Geometry: see drawing. Coordinates: mm, zero at the bounding-box minimum. A direction names the side the tool comes from. Round coordinates to 2 decimals unless told otherwise and drop trailing zeros. Write each loop counter-clockwise with the first axis right and the second up, starting at its lowest first coordinate (ties: lowest second). Pieces come first, ordered by that corner, then holes. Notation, with made-up numbers: M 13,-20 L 17,-20 A30 cw 17,13 Z; hole C 55,-13.75 d8. An arc over 180 degrees is marked long. Use one line per item in the form item = value. Start each with the question number.
Item 1: Section query D-D (y = 5.5). Return loops of the section in (x, z) (1 decimal), and give its area (3 significant figures).
Item 2: Pin query (flat end, axial travel): pin 1 Ø1.5 at (y, z) = (10.5, 0.5) entering from -X (1 decimal); pin 2 Ø1 at (y, z) = (31, 1) entering from -X. Return the tip coordinate at first contact, or that it passes through.
Item 3: Section query B-B (x = 26). Return loops of the section in (y, z), and give its area (3 significant figures).
Item 4: Section query A-A (y = 35.1). Return loops of the section in (x, z) (1 decimal).
Item 5: Pull-direction query (X, two-part tool) for the marked faces 3, 4 and 5; classes: pulls with the +X half, pulls with the -X half, needs draft (parallel to the pull), parting line crosses it, or undercut.
Item 6: Reachability of the marked faces 1 and 2 from +Z, -Z, +X, -X, +Y, -Y: full face, straight path, thin tool, end or side. Return the list, or none.
Item 7: Ray query, probe 1 along Y at (x, z) = (12, 1.5) (1 decimal); probe 2 along Y at (x, z) = (14, 0.95); probe 3 along X at (y, z) = (22.5, 1.35). Return the intervals inside material, ascending.
Item 8: Section query C-C (z = 0.9). Return loops of the section in (x, y).
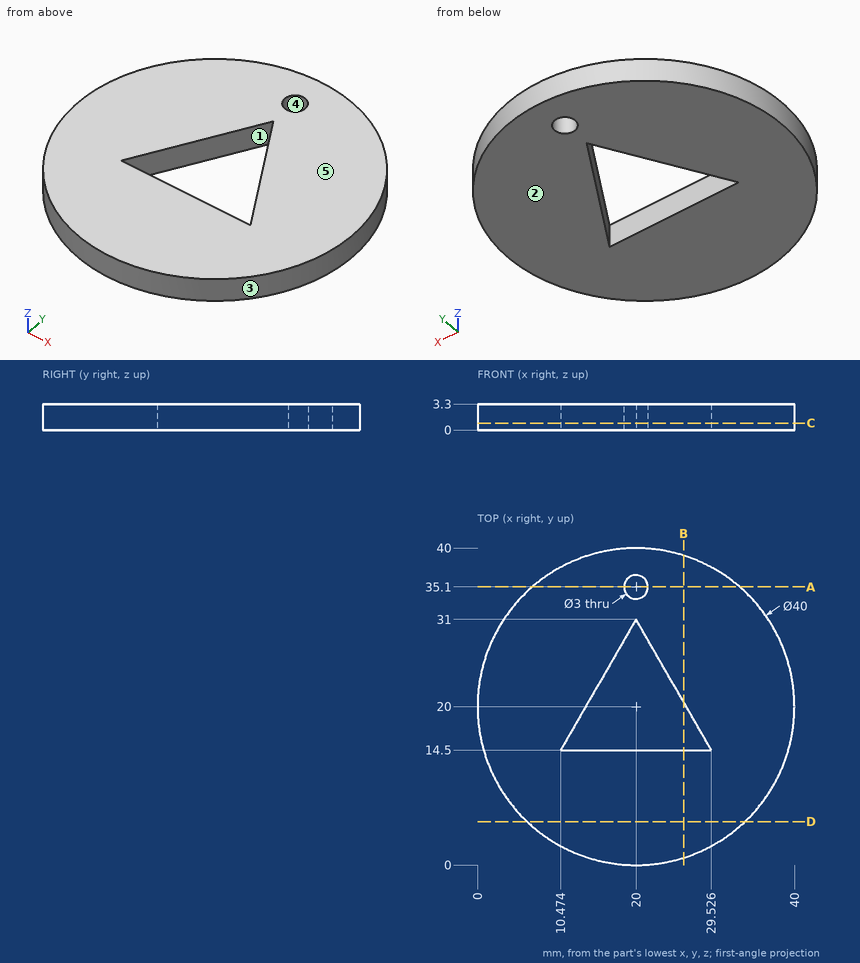
Working result:
q1.outline = M 6.2,0 L 33.8,0 L 33.8,3.3 L 6.2,3.3 Z
q1.area = 90.9 mm²
q2.pin_1 = 2
q2.pin_2 = 2.98
q3.outline = M 0.92,0 L 14.5,0 L 14.5,3.3 L 0.92,3.3 Z; M 20.61,0 L 39.08,0 L 39.08,3.3 L 20.61,3.3 Z
q3.area = 106 mm²
q4.outline = M 6.9,0 L 18.5,0 L 18.5,3.3 L 6.9,3.3 Z; M 21.5,0 L 33.1,0 L 33.1,3.3 L 21.5,3.3 Z
q5.face_3 = parting line crosses it
q5.face_4 = undercut
q5.face_5 = needs draft
q6.face_1 = +Z, -Z
q6.face_2 = -Z, +X, -X, +Y, -Y
q7.probe_1 = 1.7 to 14.5, 17.1 to 38.3
q7.probe_2 = 0.92 to 14.5, 20.61 to 39.08
q7.probe_3 = 0.16 to 15.09, 24.91 to 39.84
q8.outline = C 20,20 d40; hole M 10.47,14.5 L 29.53,14.5 L 20,31 Z; hole C 20,35.1 d3
